from build123d import *

# Parameters (mm, degrees)
SKETCH1_W           = 25
SKETCH1_H           = 30
BOSS_EXTRUDE1_DEPTH = 2
SKETCH2_W           = 25
SKETCH2_H           = 15
BOSS_EXTRUDE2_DEPTH = 18
SKETCH3_R           = 6
CUT_EXTRUDE1_DEPTH  = 36.355339059
SKETCH4_R           = 2
CUT_EXTRUDE2_DEPTH  = 28.950849719
SKETCH5_R           = 2
CUT_EXTRUDE3_DEPTH  = 27.556543565


with BuildPart() as part:
    # Sketch1 → Boss-Extrude1 (new body)
    with BuildSketch(Plane(origin=(0, 0, 0), x_dir=(1, 0, 0), z_dir=(0, 1, 0))):
        Rectangle(SKETCH1_W, SKETCH1_H)
    extrude(amount=BOSS_EXTRUDE1_DEPTH)

    # Sketch2 → Boss-Extrude2 (add)
    with BuildSketch(Plane(origin=(0, 2, 0), x_dir=(1, 0, 0), z_dir=(0, 1, 0))):
        Rectangle(SKETCH2_W, SKETCH2_H)
    extrude(amount=BOSS_EXTRUDE2_DEPTH)

    # Sketch3 → Cut-Extrude1 (cut, through all)
    with BuildSketch(Plane.ZY.offset(12.5)):
        with Locations((0, 11)):
            Circle(SKETCH3_R)
    extrude(amount=-CUT_EXTRUDE1_DEPTH, mode=Mode.SUBTRACT)

    # Sketch4 → Cut-Extrude2 (cut, through all)
    with BuildSketch(Plane(origin=(0, 20, 0), x_dir=(1, 0, 0), z_dir=(0, 1, 0))):
        with Locations(Location((0, 0, 0), (0, 0, 270))):
            Circle(SKETCH4_R)
    extrude(amount=-CUT_EXTRUDE2_DEPTH, mode=Mode.SUBTRACT)

    # Sketch5 → Cut-Extrude3 (cut, through all)
    with BuildSketch(Plane(origin=(0, 2, 0), x_dir=(1, 0, 0), z_dir=(0, 1, 0))):
        with Locations(Location((0, 11.25, 0), (0, 0, 270))):
            Circle(SKETCH5_R)
        with Locations(Location((0, -11.25, 0), (0, 0, 90))):
            Circle(SKETCH5_R)
    extrude(amount=-CUT_EXTRUDE3_DEPTH, mode=Mode.SUBTRACT)


solid = part.part
Check sheet for the modelled part. Datum: model origin and axes. Units: mm. A direction names the side the tool comes from. Coordinates: 2 decimals unless noted, no trailing zeros. Loops run counter-clockwise (first coordinate to the right, second up) from the corner with the lowest first, then second, coordinate; pieces in that order, holes last. Notation, with made-up numbers: (47.5, -16.5) -> (106.5, -16.5) arc R12 ccw to (106.5, -7.5) -> close; hole circle Ø4 at (-40, 65). An arc over 180 degrees is marked (long way). Answer in a Markdown table with one row per item.
1. Sectioned sample at A-A, the plane z = 11.25. Record the boundary of the cut face in (x, y).
Check values:
| item | result |
|---|---|
| outline | (-12.5, 0) -> (-2, 0) -> (-2, 2) -> (-12.5, 2) -> close; (2, 0) -> (12.5, 0) -> (12.5, 2) -> (2, 2) -> close |
2. Release check for a two-part mould opening along Z. For faces 1 (the face through (0, 11, 7.5)), 2 (the face through (0, 18, -2)), 3 (the face through (-3, 20, 0)) record: released by +Z, released by -Z, zero draft, split by the parting line, or undercut.
Check values:
| item | result |
|---|---|
| face 1 | released by +Z |
| face 2 | undercut |
| face 3 | zero draft |
3. Material ranges on line 1 along Z through (x, y) = (0, 3.2); line 2 along Y through (x, z) = (-4.25, 0); line 3 along X through (y, z) = (0.7, -11.25), recorded low to high. Write a range as [from, to].
Check values:
| item | result |
|---|---|
| line 1 | z = [-7.5, -2], [2, 7.5] |
| line 2 | y = [0, 5], [17, 20] |
| line 3 | x = [-12.5, -2], [2, 12.5] |
4. Sectioned sample at D-D, the plane y = 11. Record the boundary of the cut face in (x, z), then the cut area to 3 significant figures.
Check values:
| item | result |
|---|---|
| outline | (-12.5, -7.5) -> (12.5, -7.5) -> (12.5, -6) -> (-12.5, -6) -> close; (-12.5, 6) -> (12.5, 6) -> (12.5, 7.5) -> (-12.5, 7.5) -> close |
| area | 75.0 mm2 |
5. Sectioned sample at B-B, the plane x = 0. Record the boundary of the cut face in (y, z).
Check values:
| item | result |
|---|---|
| outline | (0, -15) -> (2, -15) -> (2, -13.25) -> (0, -13.25) -> close; (0, -9.25) -> (2, -9.25) -> (2, -7.5) -> (20, -7.5) -> (20, -2) -> (16.66, -2) arc R6 cw to (5.34, -2) -> (0, -2) -> close; (0, 2) -> (5.34, 2) arc R6 cw to (16.66, 2) -> (20, 2) -> (20, 7.5) -> (2, 7.5) -> (2, 9.25) -> (0, 9.25) -> close; (0, 13.25) -> (2, 13.25) -> (2, 15) -> (0, 15) -> close |
6. Sectioned sample at C-C, the plane y = 1.5. Record the boundary of the cut face in (x, z).
Check values:
| item | result |
|---|---|
| outline | (-12.5, -15) -> (12.5, -15) -> (12.5, 15) -> (-12.5, 15) -> close; hole circle Ø4 at (0, -11.25); hole circle Ø4 at (0, 0); hole circle Ø4 at (0, 11.25) |
7. Access from +Z, -Z, +X, -X, +Y, -Y to the whole of each face (thin tool, end or side, straight path). Record for faces 4 (the face through (0, 2, 9)), 5 (the face through (-1.217, 1.014, -12.837)), 6 (the face through (0, 2, -14)).
Check values:
| item | result |
|---|---|
| face 4 | +Z, +X, -X, +Y |
| face 5 | +Y, -Y |
| face 6 | -Z, +X, -X, +Y |
8. Go/stop test with flat-tipped pins: pin 1 (3 mm diameter, centred on x = 0, z = -11.25, fed in from +Y); pin 2 (2 mm diameter, centred on x = -2.5, z = 11, fed in from +Y); pin 3 (9 mm diameter, centred on x = 5, y = 15.5, fed in from +Z); pin 4 (9 mm diameter, centred on x = -1, y = 9, fed in from -Z). Record where each tip stops, or that it passes through.
Check values:
| item | result |
|---|---|
| pin 1 | passes through |
| pin 2 | stops at y = 2 |
| pin 3 | stops at z = 7.5 |
| pin 4 | stops at z = -7.5 |
